```python
from build123d import *

# Parameters (mm, degrees)
SKETCH1_R                = 2.5
BOSS_EXTRUDE1_DEPTH      = 2
FILLET1_R                = 10
FILLET2_R                = 10
BOSS_EXTRUDE2_DEPTH      = 5.3
BOSS_EXTRUDE2_DEPTH_BACK = 4.5
FILLET7_R                = 2
FILLET8_R                = 2


with BuildPart() as part:
    # Sketch1 → Boss-Extrude1 (new body)
    with BuildSketch(Plane(origin=(0, 0, 0), x_dir=(1, 0, 0), z_dir=(0, 1, 0))):
        with BuildLine():
            Line((4.734439188, 4.337505525), (-11.123424173, -8.60036928))
            Line((-11.123424173, -8.60036928), (-1.31921636, -8.60036928))
            Line((-1.31921636, -8.60036928), (10.297086052, 1.061724594))
            Line((10.297086052, 1.061724594), (13.693514413, 10.480195617))
            ThreePointArc((13.693514413, 10.480195617), (12.643820806, 18.747230765), (7.611903427, 12.10452542))
            Line((7.611903427, 12.10452542), (4.734439188, 4.337505525))
        make_face()
        with Locations(Location((11.482625797, 14.39963072, 0), (0, 0, 270))):
            Circle(SKETCH1_R, mode=Mode.SUBTRACT)
    extrude(amount=BOSS_EXTRUDE1_DEPTH)

    # Fillet1
    fillet1_edges = [part.edges().sort_by_distance(p)[0] for p in [
        (10.297086052, 1, -1.061724594),
    ]]
    fillet(fillet1_edges, radius=FILLET1_R)

    # Fillet2
    fillet2_edges = [part.edges().sort_by_distance(p)[0] for p in [
        (4.734439188, 1, -4.337505525),
    ]]
    fillet(fillet2_edges, radius=FILLET2_R)

    # Sketch6 → Boss-Extrude2 (add, two sides: drawn at the far end of the back side and taken through both)
    with BuildSketch(Plane(origin=(-6.65, 0, 0), x_dir=(0, 0, -1), z_dir=(1, 0, 0)).offset(-BOSS_EXTRUDE2_DEPTH_BACK)):
        Polygon((-8.60036928, 2.725), (-6.60036928, 2), (-6.60036928, 0), (-8.60036928, -0.725), align=None)
    extrude(amount=BOSS_EXTRUDE2_DEPTH + BOSS_EXTRUDE2_DEPTH_BACK)

    # Fillet7
    fillet7_edges = [part.edges().sort_by_distance(p)[0] for p in [
        (6.646109692, 0, -9.497598443),
        (4.438286722, 0, -4.549211293),
        (-3.023640286, 0, 1.992039552),
        (12.456410034, 0, -7.049641368),
        (9.999920903, 0, -1.270100821),
        (3.443902415, 0, 4.638549149),
    ]]
    fillet(fillet7_edges, radius=FILLET7_R - 0.0001)  # a hair under: the kernel refuses the full size

    # Fillet8
    fillet8_edges = [part.edges().sort_by_distance(p)[0] for p in [
        (12.744313914, 0, -18.719137995),
    ]]
    fillet(fillet8_edges, radius=FILLET8_R - 0.0001)  # a hair under: the kernel refuses the full size


solid = part.part
```
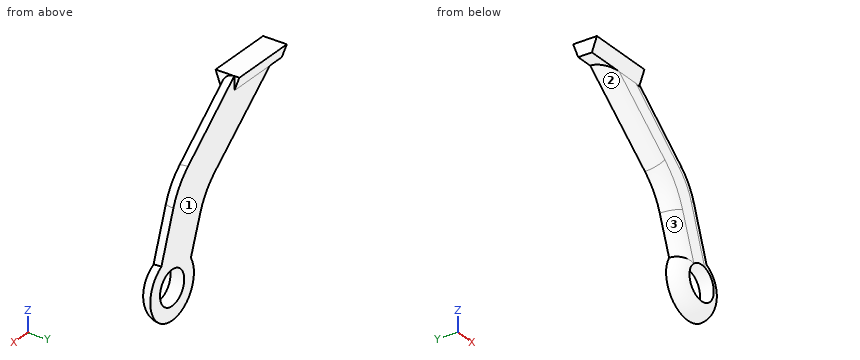
Read the model definition and answer for the solid it produces. Units are mm, in the model's axes. Face numbers are marked on the shaded views. Give positions to 0.01 mm unless a question says otherwise; leave off trailing zeros. Write each loop counter-clockwise with the first axis right and the second up, starting at its lowest first coordinate (ties: lowest second). Pieces come first, ordered by that corner, then holes. Notation, with made-up numbers: (9.25, 10) -> (14.25, 10) arc R19 cw to (14.25, 46) -> close; hole circle Ø11 at (44.25, 68). An arc over 180 degrees is marked (long way). Answer as a JSON object with one key per item and string values.
1) Section A-A on y = 0.8 is taken. Write down the section's boundary in (x, z), then the cut area to 3 significant figures.
Findings below:
{"outline": "(-11.15, 6.6) -> (-8.04, 6.6) -> (2.88, -2.31) arc R10.4 cw to (6.06, -6.75) -> (8.06, -12.15) arc R4.1 ccw (long way) to (13.37, -10.76) -> (10.84, -3.75) arc R9.6 ccw to (7.95, 0.37) -> (-1.35, 8.11) -> (-1.35, 8.6) -> (-11.15, 8.6) -> close; hole circle Ø5 at (11.48, -14.4)", "area": "180 mm^2"}
2) For a pull along Z with two mould halves and no side action, classify the marked faces 1, 2 and 3 as pulls with the +Z half, pulls with the -Z half, needs draft (parallel to the pull), parting line crosses it, or undercut.
Findings below:
{"face 1": "needs draft", "face 2": "pulls with the -Z half", "face 3": "undercut"}
3) Straight lines are drawn through the part: probe 1 along Y at (x, z) = (9, -9.25); probe 2 along X at (y, z) = (1.8, -16.25); probe 3 along X at (y, z) = (0.8, -16.25). For each, find the intervals that lie inside material, in ascending order. Write a range as from..to.
Findings below:
{"probe 1": "y = 0..2", "probe 2": "x = 7.39..9.8, 13.16..15.57", "probe 3": "x = 7.82..9.8, 13.16..15.14"}
4) Flat-ended cylindrical pins translate along their axes: pin 1 Ø6.5 at (x, z) = (11.48, -14.4) entering from -Y; pin 2 Ø1 at (x, y) = (-9, 1) entering from -Z; pin 3 Ø1.5 at (x, z) = (11, 1.5) entering from +Y; pin 4 Ø1.7 at (y, z) = (0.5, 8) entering from +X. Find the tip coordinate at first contact, or state that the pin passes through.
Findings below:
{"pin 1": "stops at y = 0", "pin 2": "stops at z = 6.6", "pin 3": "passes through", "pin 4": "stops at x = -0.19"}
